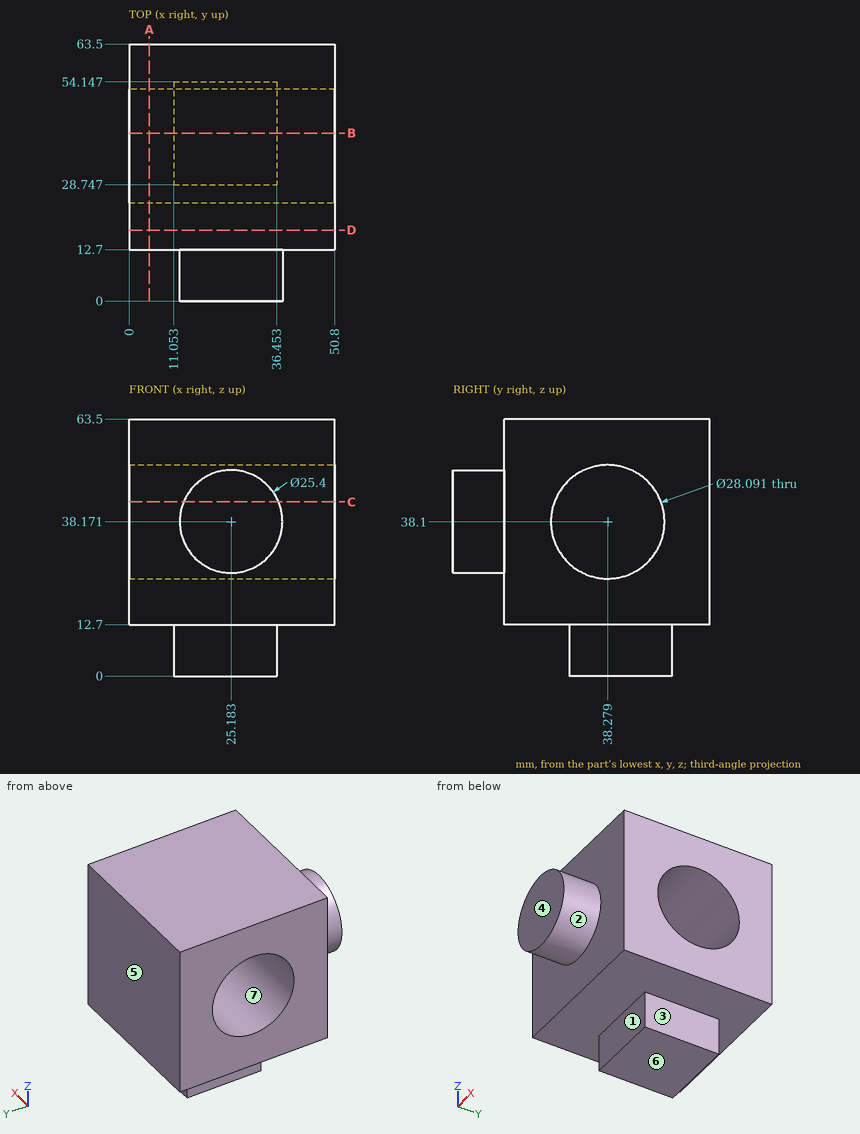
Geometry check sheet. Reference: drawing and pictorial views, mm from the part's lowest x, y, z. A direction names the side the tool comes from. Coordinates: 2 decimals unless noted, no trailing zeros. Write each loop counter-clockwise with the first axis right and the second up, starting at its lowest first coordinate (ties: lowest second). Pieces come first, ordered by that corner, then holes. Notation, with made-up numbers: M 88.5,22.25 L 139.5,22.25 A24 ccw 139.5,58.25 Z; hole C -22,-37.75 d10. An arc over 180 degrees is marked long. One line per question, with ' | ' between items.
1) Sectioned sample at B-B on y = 41.5. Record the cut outline in (x, z), then the cut area to 3 significant figures.
Solutions:
outline: M 0,12.7 L 11.05,12.7 L 11.05,0 L 36.45,0 L 36.45,12.7 L 50.8,12.7 L 50.8,24.43 L 0,24.43 Z; M 0,51.77 L 50.8,51.77 L 50.8,63.5 L 0,63.5 Z | area: 1,510 mm^2
2) Access from +Z, -Z, +X, -X, +Y, -Y to the whole of each face (thin tool, end or side, straight path). Record for the marked faces 1, 2 and 3.
Solutions:
face 1: -Z, +X, -X, -Y | face 2: -Y | face 3: -Z, +X, +Y, -Y
3) Depth check by flat-ended pin: pin 1 Ø6.5 at (x, z) = (27, 6) entering from -Y; pin 2 Ø8 at (x, y) = (16, 22) entering from -Z; pin 3 Ø3 at (y, z) = (45.5, 8) entering from +X. Enter the tip coordinate at first touch or a pass-through.
Solutions:
pin 1: y = 28.75 | pin 2: z = 12.7 | pin 3: x = 36.45
4) Sectioned sample at C-C on z = 43. Record the cut outline in (x, y) (1 decimal).
Solutions:
outline: M 0,12.7 L 13.4,12.7 L 13.4,0 L 36.9,0 L 36.9,12.7 L 50.8,12.7 L 50.8,25.1 L 0,25.1 Z; M 0,51.4 L 50.8,51.4 L 50.8,63.5 L 0,63.5 Z
5) Sectioned sample at D-D on y = 17.5. Record the cut outline in (x, z).
Solutions:
outline: M 0,12.7 L 50.8,12.7 L 50.8,63.5 L 0,63.5 Z
6) Release check for a two-part mould opening along Y. For the marked faces 4, 5, 6 and 7 record: +Y half, -Y half, draft (parallel to the pull), parting line (faces both ways), or undercut.
Solutions:
face 4: -Y half | face 5: +Y half | face 6: draft | face 7: undercut
7) Material ranges on L1, parallel to Y at x = 28, z = 38; L2, parallel to Y at x = 45.5, z = 15; L3, parallel to X at y = 43.5, z = 7, recorded low to high.
Solutions:
L1: 0 to 24.23, 52.32 to 63.5 | L2: 12.7 to 63.5 | L3: 11.05 to 36.45
8) Sectioned sample at A-A on x = 5. Record the cut outline in (y, z) (1 decimal), then the cut area to 3 significant figures.
Solutions:
outline: M 12.7,12.7 L 63.5,12.7 L 63.5,63.5 L 12.7,63.5 Z; hole C 38.3,38.1 d28.1 | area: 1,960 mm^2
